Input: part model. Units: mm. Frame: model coordinates. Coordinates: 2 decimals unless noted, no trailing zeros. Loops run counter-clockwise (first coordinate to the right, second up) from the corner with the lowest first, then second, coordinate; pieces in that order, holes last.
```python
from build123d import *

# Parameters (mm, degrees)
F0_W      = 150.0115171075
F0_H      = 150.0115022063
F1_DEPTH  = 50
F2_DEPTH  = 50
F3_T      = -5
F4_W      = 50.3282439895
F4_H      = 50.0862784684
F5_DEPTH  = 50
F6_R      = 25.7006976181
F7_DEPTH  = 50
F9_DEPTH  = 50
F11_DEPTH = 50
F12_W     = 13.2862403989
F12_H     = 45.7488838583
F13_DEPTH = 50
F15_DEPTH = 50
F17_DEPTH = 50


with BuildPart() as f1:
    # F0 (on Front) → F1 (new body)
    with BuildSketch(Plane.XZ):
        with Locations((0.1207850873, -0.2415664494)):
            Rectangle(F0_W, F0_H)
    extrude(amount=F1_DEPTH)

    # F2 (add): a face of the model
    f2_faces = [f1.faces().sort_by_distance(p)[0] for p in [
        (0.1207850873, 0, -0.2415664494),
    ]]
    extrude(f2_faces, amount=F2_DEPTH)

    # F3
    f3_openings = [f1.faces().sort_by_distance(p)[0] for p in [
        (0.120785, -50, -0.241566),
    ]]
    offset(amount=F3_T, openings=f3_openings)

    # F4 (on face) → F5 (join)
    with BuildSketch(Plane.XZ.offset(-45)):
        with Locations((-21.2294475641, 41.4939280599)):
            Rectangle(F4_W, F4_H)
    extrude(amount=F5_DEPTH)

    # F6 (on face) → F7 (join)
    with BuildSketch(Plane.XZ.offset(-45)):
        with Locations((34.225974232, 41.3267239928)):
            Circle(F6_R)
    extrude(amount=F7_DEPTH)

    # F8 (on face) → F9 (join)
    with BuildSketch(Plane.XZ.offset(-45)):
        Polygon((-25.8233335135, -36.9013702446), (-60.1888511064, -13.4322265214), (-63.3309669793, -54.9282096326), align=None)
    extrude(amount=F9_DEPTH)

    # F10 (on face) → F11 (join)
    with BuildSketch(Plane.XZ.offset(-45)):
        Polygon((32.4785027368, -35.1417758495), (17.0084361272, -12.288266328), (-9.5070565099, -19.9390511614), (-10.4244655785, -47.5210057505), (15.5240370727, -56.9168063293), align=None)
    extrude(amount=F11_DEPTH)

    # F12 (on face) → F13 (join)
    with BuildSketch(Plane.XZ.offset(-45)):
        with Locations((-59.0873472393, 40.5877782032)):
            Rectangle(F12_W, F12_H)
    extrude(amount=F13_DEPTH)

    # F14 (on face) → F15 (join)
    with BuildSketch(Plane.XZ.offset(-45)):
        Polygon((-49.7810505331, 0), (-32.3597341776, -20.085580647), (-7.4375732802, -16.9400647283), (-21.7133741826, 0), align=None)
    extrude(amount=F15_DEPTH)

    # F16 (on face) → F17 (join)
    with BuildSketch(Plane.XZ.offset(-45)):
        with BuildLine():
            add(Edge.make_bspline(
                [(44.1004857421, -25.8926860988), (32.8076134685, -26.462876483), (5.9337500795, 8.9077984279), (73.1779523154, 9.3996996285), (54.7857295651, -25.3531755887), (44.1004857421, -25.8926860988)],
                knots=[0, 0, 0, 0, 0.3375027868, 0.6806570126, 1, 1, 1, 1], degree=3))
        make_face()
    extrude(amount=F17_DEPTH)


solid = f1.part
```
Item 1: Line query: L1, parallel to Z at x = 41, y = -36; L2, parallel to X at y = 2.5, z = -0.5; L3, parallel to X at y = -31, z = -39.5. Output: solid intervals per line, ascending.
Result:
L1: z = -75.25 to -70.25, 69.76 to 74.76
L2: x = -74.88 to -69.88, -49.35 to -21.29, 23.79 to 58.21, 70.13 to 75.13
L3: x = -74.88 to -69.88, 70.13 to 75.13
Item 2: Section query C-C (z = 61). Output: boundary loops of the cut face in (x, y).
Result:
outline: (-74.88, -50) - (-69.88, -50) - (-69.88, 45) - (-65.73, 45) - (-65.73, -5) - (-52.44, -5) - (-52.44, 45) - (-46.39, 45) - (-46.39, -5) - (3.93, -5) - (3.93, 45) - (17.69, 45) - (17.69, -5) - (50.76, -5) - (50.76, 45) - (70.13, 45) - (70.13, -50) - (75.13, -50) - (75.13, 50) - (-74.88, 50) - close
Item 3: Section query A-A (y = -28). Output: boundary loops of the cut face in (x, z), then the cut area to 3 significant figures.
Result:
outline: (-74.88, -75.25) - (75.13, -75.25) - (75.13, 74.76) - (-74.88, 74.76) - close; hole (-69.88, -70.25) - (70.13, -70.25) - (70.13, 69.76) - (-69.88, 69.76) - close
area: 2,900 mm2
Item 4: Section query B-B (x = -29.5). Output: boundary loops of the cut face in (y, z), then the cut area to 3 significant figures.
Result:
outline: (-50, -75.25) - (50, -75.25) - (50, 74.76) - (-50, 74.76) - (-50, 69.76) - (45, 69.76) - (45, 66.54) - (-5, 66.54) - (-5, 16.45) - (45, 16.45) - (45, 0) - (-5, 0) - (-5, -19.72) - (45, -19.72) - (45, -34.39) - (-5, -34.39) - (-5, -38.67) - (45, -38.67) - (45, -70.25) - (-50, -70.25) - close
area: 5,400 mm2
Item 5: Contact query for flat-ended pins moving along their axis: P1, Ø21.5, axis at x = 5.5, z = -26.5, coming from the -Y side; P2, Ø4, axis at x = -19.5, z = -52.5, coming from the -Y side. Output: stop coordinate, or through.
Result:
P1: stops at y = -5
P2: stops at y = 45
Item 6: Mould query, pull axis Z, two halves, no side actions, for faces 1 (the face through (-1, 50, 1)), 2 (the face through (-1, -1, -75.247)), 3 (the face through (-36, 20, 0)). Classes: +Z half, -Z half, draft (parallel to the pull), parting line (faces both ways), or undercut.
Result:
face 1: draft
face 2: -Z half
face 3: undercut
Item 7: Section query D-D (y = 11). Count the separate pieces of the cut face and the enclosed holes in it, then the cut area to 3 significant figures.
Result:
separate pieces: 8
enclosed holes: 1
area: 11,600 mm2
